Part model, mm, in its own coordinate system. A direction names the side the tool comes from. Round coordinates to 2 decimals unless told otherwise and drop trailing zeros. Write each loop counter-clockwise with the first axis right and the second up, starting at its lowest first coordinate (ties: lowest second). Pieces come first, ordered by that corner, then holes. Notation, with made-up numbers: (63, -40) -> (102, -40) arc R24 ccw to (102, -9) -> close; hole circle Ø11 at (89, 68). An arc over 180 degrees is marked (long way). Return JSON: item names as keys, results as strings. Group by question number.
(1) Drop flat-ended pins along their axis: pin 1 Ø2 at (x, y) = (-47, -24.5) entering from +Z; pin 2 Ø1 at (y, z) = (-16, 16.5) entering from -X; pin 3 Ø5 at (x, y) = (-35, -13) entering from +Z; pin 4 Ø4 at (x, z) = (-26, 47.5) entering from +Y. Give the stop position or say it passes through.
(2) Drill centre lines: L1, parallel to X at y = -12, z = 30; L2, parallel to X at y = -15, z = 25.5; L3, parallel to X at y = -16, z = 15. Where is each one in solid material? Low to high. Write a range as from..to.
(3) Mould opens along Z. For faces 3 (the flat face through (-33.135, -20, 25)), 4 (the flat face through (-14, -15.773, 25)), 5 (the cylindrical face through (20.11, -7.78, 24.29)) say: +Z half, -Z half, draft (parallel to the pull), parting line (faces both ways), or undercut.
(4) Saw through at D-D (x = -13). List the corners of the cut face in (y, z), plus the area to 3 significant figures.
(5) Tool access for faces 1 (the flat face through (-21.35, -7.78, 48.03)), 2 (the flat face through (-36, -20, 19.833)): list every direction of +Z, -Z, +X, -X, +Y, -Y with a clear straight run to the whole face (end or side of a thin tool).
(6) Saw through at A-A (x = 6). List the corners of the cut face in (y, z).
(7) Saw through at C-C (z = 23). State how many separate pieces and enclosed holes the cut face has, plus the area to 3 significant figures.
from build123d import *

# Parameters (mm, degrees)
F0_R     = 10.16
F1_DEPTH = 15.7734
F2_DEPTH = 40.2336
F3_R     = 3.302


with BuildPart() as f1:
    # F0 (on Front) → F1 (new body)
    with BuildSketch(Plane.XZ):
        with BuildLine():
            ThreePointArc((-47.867193, 52.785754), (-30.993815, 42.995474), (-24.33484, 24.659213))
            ThreePointArc((-24.33484, 24.659213), (-30.993815, 6.322951), (-47.867193, -3.467329))
            Line((-47.867193, -3.467329), (4.426925, 5.908185))
            ThreePointArc((4.426925, 5.908185), (20.11516, 24.659213), (4.426925, 43.41024))
            Line((4.426925, 43.41024), (-47.867193, 52.785754))
        make_face()
        with Locations((1.06516, 24.659213)):
            Circle(F0_R, mode=Mode.SUBTRACT)
    extrude(amount=F1_DEPTH)

    # F0 (on Front) → F2 (join)
    with BuildSketch(Plane.XZ):
        with BuildLine():
            ThreePointArc((-47.867193, -3.467329), (-30.993815, 6.322951), (-24.33484, 24.659213))
            ThreePointArc((-24.33484, 24.659213), (-30.993815, 42.995474), (-47.867193, 52.785754))
            ThreePointArc((-47.867193, 52.785754), (-81.48484, 24.659213), (-47.867193, -3.467329))
        make_face()
        with BuildLine():
            ThreePointArc((-39.462075, 19.833213), (-67.19734, 24.659213), (-39.462075, 29.485213))
            Line((-39.462075, 29.485213), (-33.135355, 29.485213))
            Line((-33.135355, 29.485213), (-33.135355, 24.659213))
            Line((-33.135355, 24.659213), (-33.135355, 19.833213))
            Line((-33.135355, 19.833213), (-39.462075, 19.833213))
        make_face(mode=Mode.SUBTRACT)
    extrude(amount=F2_DEPTH)

    # F3
    f3_edges = [f1.edges().sort_by_distance(p)[0] for p in [
        (-57.952487, -40.2336, 52.785754),
    ]]
    fillet(f3_edges, radius=F3_R)


solid = f1.part
Computed values:
{
 "1": {"pin 1": "z = 52.81", "pin 2": "x = -80.44", "pin 3": "z = 50.93", "pin 4": "y = 0"},
 "2": {"L1": "-80.98..-66.16, -39.66..-7.58, 9.71..19.35", "L2": "-81.47..-67.17, -33.14..-9.06, 11.19..20.1", "L3": "-79.8..-63.44, -42.38..-26.02"},
 "3": {"face 3": "undercut", "face 4": "draft", "face 5": "parting line"},
 "4": {"outline": "(-15.77, 2.78) -> (0, 2.78) -> (0, 46.53) -> (-15.77, 46.53) -> close", "area": "690 mm2"},
 "5": {"face 1": "+Z, +X, +Y, -Y", "face 2": "+Y, -Y"},
 "6": {"outline": "(-15.77, 6.26) -> (0, 6.26) -> (0, 15.78) -> (-15.77, 15.78) -> close; (-15.77, 33.54) -> (0, 33.54) -> (0, 43.06) -> (-15.77, 43.06) -> close"},
 "7": {"separate pieces": "3", "enclosed holes": "0", "area": "1,310 mm2"}
}
